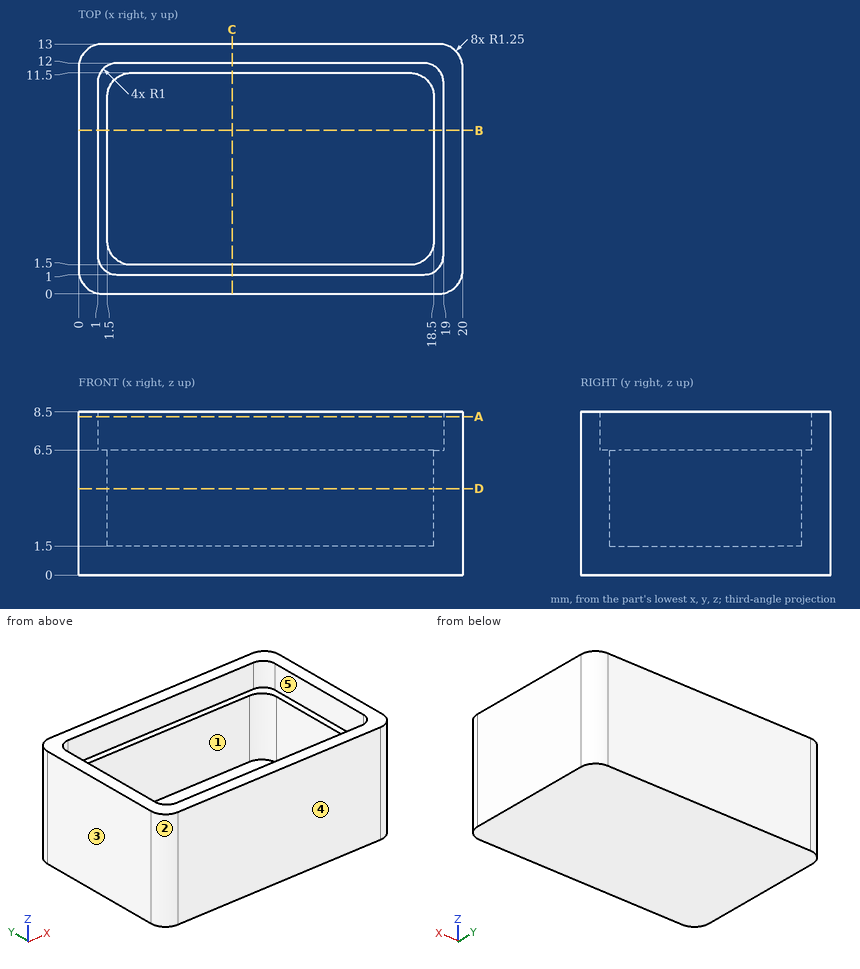
Job drawing, mm, ordinate dimensions from the low corner. One solid piece. A direction names the side the tool comes from. Give positions to 0.01 mm unless a question says otherwise; leave off trailing zeros. Write each loop counter-clockwise with the first axis right and the second up, starting at its lowest first coordinate (ties: lowest second). Pieces come first, ordered by that corner, then holes. Notation, with made-up numbers: M 18.5,-8 L 48.5,-8 A21 cw 48.5,12 Z; hole C 26,8.25 d6. An arc over 180 degrees is marked long. One line per item, written item: value. Start each with the question number.
Q1. Saw through at A-A, the plane z = 8.25. Write the cut outline in (x, y).
Q2. Two-plate mould, pull along Y, no slides. Class the marked faces 3, 4 and 5: +Y half, -Y half, draft (parallel to the pull), parting line (faces both ways), or undercut.
Q3. Drop flat-ended pins along their axis: pin 1 Ø5.5 at (x, y) = (8.5, 7) entering from +Z; pin 2 Ø1 at (y, z) = (4.5, 7) entering from -X. Give the stop position or say it passes through.
Q4. Saw through at D-D, the plane z = 4.5. Write the cut outline in (x, y).
Q5. Saw through at C-C, the plane x = 8. Write the cut outline in (y, z).
Q6. Saw through at B-B, the plane y = 8.5. Write the cut outline in (x, z).
Q7. 3-axis set-ups, long thin cutter, end or side, ignore diameter. For the marked faces 1 and 2: which of +Z, -Z, +X, -X, +Y, -Y reach the whole face in a straight line?
Q8. Probe probe 1 along Y at (x, z) = (2.75, 6.75); probe 2 along X at (y, z) = (7.75, 2.75); probe 3 along Y at (x, z) = (4.25, 2). List the from-to ranges inside material, lowest first. Write a range as [from, to].
Output values:
1. outline: M 0,1.25 A1.25 ccw 1.25,0 L 18.75,0 A1.25 ccw 20,1.25 L 20,11.75 A1.25 ccw 18.75,13 L 1.25,13 A1.25 ccw 0,11.75 Z; hole M 1,2 A1 ccw 2,1 L 18,1 A1 ccw 19,2 L 19,11 A1 ccw 18,12 L 2,12 A1 ccw 1,11 Z
2. face 3: draft
2. face 4: -Y half
2. face 5: undercut
3. pin 1: stops at z = 1.5
3. pin 2: stops at x = 0
4. outline: M 0,1.25 A1.25 ccw 1.25,0 L 18.75,0 A1.25 ccw 20,1.25 L 20,11.75 A1.25 ccw 18.75,13 L 1.25,13 A1.25 ccw 0,11.75 Z; hole M 1.5,2.75 A1.25 ccw 2.75,1.5 L 17.25,1.5 A1.25 ccw 18.5,2.75 L 18.5,10.25 A1.25 ccw 17.25,11.5 L 2.75,11.5 A1.25 ccw 1.5,10.25 Z
5. outline: M 0,0 L 13,0 L 13,8.5 L 12,8.5 L 12,6.5 L 11.5,6.5 L 11.5,1.5 L 1.5,1.5 L 1.5,6.5 L 1,6.5 L 1,8.5 L 0,8.5 Z
6. outline: M 0,0 L 20,0 L 20,8.5 L 19,8.5 L 19,6.5 L 18.5,6.5 L 18.5,1.5 L 1.5,1.5 L 1.5,6.5 L 1,6.5 L 1,8.5 L 0,8.5 Z
7. face 1: +Z
7. face 2: +Z, -Z, -X, -Y
8. probe 1: y = [0, 1], [12, 13]
8. probe 2: x = [0, 1.5], [18.5, 20]
8. probe 3: y = [0, 1.5], [11.5, 13]
